Could you check a few things on this model? Use its own coordinates, in mm. A direction names the side the tool comes from. Coordinates: 2 decimals unless noted, no trailing zeros. Write each loop counter-clockwise with the first axis right and the second up, starting at its lowest first coordinate (ties: lowest second). Pieces come first, ordered by that corner, then holes.
```python
from build123d import *

# Parameters (mm, degrees)
SKETCH_1_R          = 4.5
EXTRUDE_1_DEPTH     = 6
SKETCH_2_R          = 6.85
CUT_EXTRUDE_1_DEPTH = 5.2
SKETCH_3_R          = 7.85
CUT_EXTRUDE_2_DEPTH = 1
SKETCH_5_R          = 6.85
CUT_EXTRUDE_3_DEPTH = 5.2
SKETCH_6_R          = 7.85
CUT_EXTRUDE_4_DEPTH = 1


with BuildPart() as part:
    # 草图1 → 凸台-拉伸1 (new body)
    with BuildSketch(Plane(origin=(0, 0, 0), x_dir=(1, 0, 0), z_dir=(0, 1, 0))):
        Polygon((-65.26232397, 5), (-70.363344484, 10), (-80.363344484, 10), (-85.26232397, 5), (-85.26232397, -5), (-80.363344484, -10), (-70.363344484, -10), (-65.26232397, -5), (72.73767603, -5), (77.636655516, -10), (87.636655516, -10), (92.739759147, -5), (92.739759147, 5), (87.636655516, 10), (77.636655516, 10), (72.73767603, 5), align=None)
        with Locations(Location((-75.363344484, 0, 0), (0, 0, 270))):
            Circle(SKETCH_1_R, mode=Mode.SUBTRACT)
        with Locations(Location((82.636655516, 0, 0), (0, 0, 270))):
            Circle(SKETCH_1_R, mode=Mode.SUBTRACT)
    extrude(amount=EXTRUDE_1_DEPTH)

    # 草图2 → 切除-拉伸1 (cut)
    with BuildSketch(Plane(origin=(0, 6, 0), x_dir=(1, 0, 0), z_dir=(0, 1, 0))):
        with Locations(Location((82.636655516, 0, 0), (0, 0, 270))):
            Circle(SKETCH_2_R)
    extrude(amount=-CUT_EXTRUDE_1_DEPTH, mode=Mode.SUBTRACT)

    # 草图3 → 切除-拉伸2 (cut)
    with BuildSketch(Plane(origin=(0, 6, 0), x_dir=(1, 0, 0), z_dir=(0, 1, 0))):
        with Locations(Location((82.636655516, 0, 0), (0, 0, 270))):
            Circle(SKETCH_3_R)
    extrude(amount=-CUT_EXTRUDE_2_DEPTH, mode=Mode.SUBTRACT)

    # 草图5 → 切除-拉伸3 (cut)
    with BuildSketch(Plane.XZ):
        with Locations(Location((-75.363344484, 0, 0), (0, 0, 270))):
            Circle(SKETCH_5_R)
    extrude(amount=-CUT_EXTRUDE_3_DEPTH, mode=Mode.SUBTRACT)

    # 草图6 → 切除-拉伸4 (cut)
    with BuildSketch(Plane.XZ):
        with Locations(Location((-75.363344484, 0, 0), (0, 0, 270))):
            Circle(SKETCH_6_R)
    extrude(amount=-CUT_EXTRUDE_4_DEPTH, mode=Mode.SUBTRACT)


solid = part.part
```
1. Please list where these lines run through material, in increasing order: line 1 along X through (y, z) = (2.1, -0.25); line 2 along X through (y, z) = (0.6, 0); line 3 along Z through (x, y) = (82, 5.5).
Verdict:
line 1: x = -85.26 to -82.21, -68.52 to 75.79, 89.48 to 92.74
line 2: x = -85.26 to -83.21, -67.51 to 78.14, 87.14 to 92.74
line 3: z = -10 to -7.82, 7.82 to 10
2. I want a section at A-A on z = 0. Please give me the cut outline in (x, y), plus the area to 3 significant figures.
Verdict:
outline: (-85.26, 0) - (-83.21, 0) - (-83.21, 1) - (-82.21, 1) - (-82.21, 5.2) - (-79.86, 5.2) - (-79.86, 6) - (-85.26, 6) - close; (-70.86, 5.2) - (-68.51, 5.2) - (-68.51, 1) - (-67.51, 1) - (-67.51, 0) - (78.14, 0) - (78.14, 0.8) - (75.79, 0.8) - (75.79, 5) - (74.79, 5) - (74.79, 6) - (-70.86, 6) - close; (87.14, 0) - (92.74, 0) - (92.74, 6) - (90.49, 6) - (90.49, 5) - (89.49, 5) - (89.49, 0.8) - (87.14, 0.8) - close
area: 907 mm2
3. I want a section at B-B on y = 3.45. Please give me the cut outline in (x, z), plus the area to 3 significant figures.
Verdict:
outline: (-85.26, -5) - (-80.36, -10) - (-70.36, -10) - (-65.26, -5) - (72.74, -5) - (77.64, -10) - (87.64, -10) - (92.74, -5) - (92.74, 5) - (87.64, 10) - (77.64, 10) - (72.74, 5) - (-65.26, 5) - (-70.36, 10) - (-80.36, 10) - (-85.26, 5) - close; hole circle Ø13.7 at (-75.36, 0); hole circle Ø13.7 at (82.64, 0)
area: 1,790 mm2
4. I want a section at C-C on x = -28. Please give me the cut outline in (y, z), plus the area to 3 significant figures.
Verdict:
outline: (0, -5) - (6, -5) - (6, 5) - (0, 5) - close
area: 60.0 mm2
5. For pin 1 (1.8 mm diameter, centred on x = 26, y = 1.5, fed in from +Z); pin 2 (3 mm diameter, centred on x = -23.5, y = 3, fed in from -Z); pin 3 (11.5 mm diameter, centred on x = -75.36, z = 0, fed in from -Y), each with a flat end and sliding along its axis, tell me the tip position at first contact or that it passes through.
Verdict:
pin 1: stops at z = 5
pin 2: stops at z = -5
pin 3: stops at y = 5.2
6. On a 3-axis mill with a long thin cutter (end or side, diameter ignored), from which of +Z, -Z, +X, -X, +Y, -Y can I reach the whole of each face in a straight line? I mean faces 5 (the face through (-83.027, 0.493, 1.702)), 6 (the face through (5, 3, -5)), 7 (the face through (3, 3, 5)), 8 (the face through (84.99, 5.51, 7.49)). Say none if no direction works.
Verdict:
face 5: -Y
face 6: -Z, +Y, -Y
face 7: +Z, +Y, -Y
face 8: +Y
7. If we mould it in two halves opening along X, with no side actions, what happens to faces 1 (the face through (75.15, 2.96, 7.46)), 2 (the face through (78.244, 0.394, -0.976)), 3 (the face through (90.224, 2.958, -7.465)), 4 (the face through (2, 6, 0))? For each: pulls with the +X half, pulls with the -X half, needs draft (parallel to the pull), parting line crosses it, or undercut.
Verdict:
face 1: undercut
face 2: undercut
face 3: pulls with the +X half
face 4: needs draft
